Check sheet for the modelled part. Datum: model origin and axes. Units: mm. A direction names the side the tool comes from. Give positions to 0.01 mm unless a question says otherwise; leave off trailing zeros. Write each loop counter-clockwise with the first axis right and the second up, starting at its lowest first coordinate (ties: lowest second). Pieces come first, ordered by that corner, then holes. Notation, with made-up numbers: M 74.25,16 L 120.25,16 A13 cw 120.25,34 Z; hole C 16,32 d1. An arc over 180 degrees is marked long. Write item = value, one per line. Start each with the question number.
1) Sectioned sample at A-A, the plane z = 2.95. Record the cut outline in (x, y).
2) Scan lines: L1, parallel to Y at x = 2, z = 2.35; L2, parallel to X at y = 78.5, z = 1.65; L3, parallel to X at y = 2, z = 1.1. Record each from-to range of solid material in increasing order.
3) Set-up check for faces 1 (the face through (-43, 1.8, 2)), 2 (the face through (-40, 82, 2)), 3 (the face through (0, 82, 2)): record each of +Z, -Z, +X, -X, +Y, -Y from which the full face is reachable in a straight line by a thin tool's end or side.
4) Gauge pin test, flat ends, axial feed: pin 1 (1.2 mm diameter, centred on y = -2.5, z = 3, fed in from -X); pin 2 (1.2 mm diameter, centred on x = -42.5, z = 3, fed in from +Y); pin 3 (0.7 mm diameter, centred on x = -43, z = 3, fed in from -Y). Record the tip position at first contact, or that the pin passes through.
Autodesk Inventor part; units mm, degrees
ref_plane "YZ Plane" through (0, 0, 0) normal (1, 0, 0) x (0, 1, 0)
ref_plane "XZ Plane" through (0, 0, 0) normal (0, 1, 0) x (-1, 0, 0)
ref_plane "XY Plane" through (0, 0, 0) normal (0, 0, 1) x (1, 0, 0)
sketch "Skizze3" plane through (0, 0, 0) normal (0, 0, 1) x (1, 0, 0)
  line L0 (0, 0) -> (-40, 0)
  line L1 (-40, 0) -> (-40, 80)
  line L2 (-40, 80) -> (0, 80)
  line L3 (0, 80) -> (0, 0)
  line L4 (-40, 78.2) -> (-45.85, 78.2)
  line L5 (-45.85, 78.2) -> (-45.85, 40)
  line L6 (-45.85, 40) -> (-40, 40)
  line L7 (-40, 40) -> (-40, 78.2)
  line L8 (-40, 80) -> (-20, 80)
  line L9 (-20, 80) -> (-20, 85.85)
  line L10 (-20, 85.85) -> (-40, 85.85)
  line L11 (-40, 85.85) -> (-40, 80)
  point P0 (-40, 40)
  point P1 (-20, 80)
  dimension "d4" = 80
  dimension "d5" = 40
  dimension "d6" = 5.85
  dimension "d7" = 1.8
  dimension "d8" = 5.85
extrude "Extrusion3" add sketch "Skizze3" along normal blind 5 contours L0 L1 L2 L3
extrude "Extrusion4" add sketch "Skizze3" along normal blind 5 contours L6 L5 L4 L1 | L2 L11 L10 L9
fillet "Rundung1" radius 2 2 edges at (-45.85, 78.2, 2.5) (-40, 85.85, 2.5)
mirror "Spiegeln1" about plane through (-45.85, 40, 0) normal (0, -1, 0) of "Extrusion4", "Rundung1"
mirror "Spiegeln2" about plane through (-20, 80, 0) normal (1, 0, 0) of "Extrusion4", "Rundung1", "Spiegeln1"
fillet "Rundung2" radius 1.5 4 edges at (0, 78.2, 2.5) (-40, 78.2, 2.5) (-40, 1.8, 2.5) (0, 1.8, 2.5)
equation "\"d6\" = d8"
properties part number "BT702_trajan20_21" material "Acryl"
Data:
q1.outline = M -45.85,3.8 A2 ccw -43.85,1.8 L -41.5,1.8 A1.5 cw -40,0.3 L -40,-3.85 A2 ccw -38,-5.85 L -2,-5.85 A2 ccw 0,-3.85 L 0,0.3 A1.5 cw 1.5,1.8 L 3.85,1.8 A2 ccw 5.85,3.8 L 5.85,76.2 A2 ccw 3.85,78.2 L 1.5,78.2 A1.5 cw 0,79.7 L 0,83.85 A2 ccw -2,85.85 L -38,85.85 A2 ccw -40,83.85 L -40,79.7 A1.5 cw -41.5,78.2 L -43.85,78.2 A2 ccw -45.85,76.2 Z
q2.L1 = 1.8 to 78.2
q2.L2 = -40.6 to 0.6
q2.L3 = -44.72 to 4.72
q3.face_1 = +Z, -Z, -X, -Y
q3.face_2 = +Z, -Z, -X, +Y
q3.face_3 = +Z, -Z, +X, +Y
q4.pin_1 = -40
q4.pin_2 = 78.2
q4.pin_3 = 1.8
